Read the model definition and answer for the solid it produces. Units are mm, in the model's axes. Coordinates: 2 decimals unless noted, no trailing zeros. Write each loop counter-clockwise with the first axis right and the second up, starting at its lowest first coordinate (ties: lowest second). Pieces come first, ordered by that corner, then holes.
1) The part is cut by section A-A (z = 0). Determine the outline of the cut face in (x, y), then the cut area to 3 significant figures.
2) The part is cut by section C-C (z = -6). Determine the outline of the cut face in (x, y).
3) Determine the mould class of faces 1 (the face through (17.996, 0.986, -18.378)), 2 (the face through (-24.397, 0.986, 12.69)), 3 (the face through (-6, 2, 6)), 4 (the face through (9.63, 0.99, -17.47)) for opening direction Z: +Z half, -Z half, draft (parallel to the pull), parting line (faces both ways), or undercut.
4) Find the intervals of material crossed by line 1 (Z direction, x = -16.5, y = 0.55); line 2 (Z direction, x = -0.5, y = 1); line 3 (Z direction, x = 9, y = 1.7), in increasing order.
5) The part is cut by section B-B (x = 0). Determine the outline of the cut face in (y, z), then the cut area to 3 significant figures.
6) The part is cut by section D-D (y = 1). Give the number of separate pieces and of enclosed holes in the cut face, then the cut area to 3 significant figures.
from build123d import *

# Parameters (mm, degrees)
SKETCH_1_R           = 27.5
EXTRUDE_1_DEPTH      = 2
SKETCH_2_R           = 8
CUT_EXTRUDE_1_DEPTH  = 39.942264957
HOLE_WIZARD_M2_1_D   = 1.6
HOLE_WIZARD_M3_4_D   = 2.5
MIRROR_2_COPY_1_D    = 2.5
HOLE_WIZARD_M2_5_1_D = 2.05


with BuildPart() as part:
    # 草图1 → 凸台-拉伸1 (new body)
    with BuildSketch(Plane(origin=(0, 0, 0), x_dir=(1, 0, 0), z_dir=(0, 1, 0))):
        with Locations(Location((0, 0, 0), (0, 0, 270))):
            Circle(SKETCH_1_R)
    extrude(amount=EXTRUDE_1_DEPTH)

    # 草图2 → 切除-拉伸1 (cut, through all)
    with BuildSketch(Plane(origin=(0, 2, 0), x_dir=(1, 0, 0), z_dir=(0, 1, 0))):
        with Locations(Location((0, 0, 0), (0, 0, 270))):
            Circle(SKETCH_2_R)
    extrude(amount=-CUT_EXTRUDE_1_DEPTH, mode=Mode.SUBTRACT)

    # M2 螺纹孔1 (through all)
    with Locations(Plane(origin=(0, 2, 0), x_dir=(1, 0, 0), z_dir=(0, 1, 0))):
        with Locations((-10, 0)):
            hole_wizard_m2_1 = Hole(HOLE_WIZARD_M2_1_D / 2)

    # M3 螺纹孔4 (through all)
    with Locations(Plane(origin=(0, 2, 0), x_dir=(1, 0, 0), z_dir=(0, 1, 0))):
        with Locations((-17.324116139, 17.324116139)):
            hole_wizard_m3_4 = Hole(HOLE_WIZARD_M3_4_D / 2)

    # 镜向1: M3 螺纹孔4 across plane
    add(hole_wizard_m3_4.mirror(Plane(origin=(0, 0, 0), x_dir=(0, 0, 1), z_dir=(1, 0, 0))), mode=Mode.SUBTRACT)

    # 镜向2: M3 螺纹孔4 across plane
    add(hole_wizard_m3_4.mirror(Plane.XY), mode=Mode.SUBTRACT)

    # 镜向2 copy 1 (through all)
    with Locations(Plane(origin=(0, 2, 0), x_dir=(-1, 0, 0), z_dir=(0, 1, 0))):
        with Locations((-17.324116139, 17.324116139)):
            Hole(MIRROR_2_COPY_1_D / 2)

    # 镜向3: M2 螺纹孔1 across plane
    add(hole_wizard_m2_1.mirror(Plane(origin=(0, 0, 0), x_dir=(0, 0, 1), z_dir=(1, 0, 0))), mode=Mode.SUBTRACT)

    # M2.5 螺纹孔1 (through all)
    with Locations(Plane(origin=(0, 2, 0), x_dir=(1, 0, 0), z_dir=(0, 1, 0))):
        with Locations((-9.497088469, 16.451681088), (9.497088469, 16.451681088)):
            hole_wizard_m2_5_1 = Hole(HOLE_WIZARD_M2_5_1_D / 2)

    # 镜向4: M2.5 螺纹孔1 across plane
    add(hole_wizard_m2_5_1.mirror(Plane.XY), mode=Mode.SUBTRACT)


solid = part.part
Reported:
1. outline: (-27.5, 0) - (-10.8, 0) - (-10.8, 2) - (-27.5, 2) - close; (-9.2, 0) - (-8, 0) - (-8, 2) - (-9.2, 2) - close; (8, 0) - (9.2, 0) - (9.2, 2) - (8, 2) - close; (10.8, 0) - (27.5, 0) - (27.5, 2) - (10.8, 2) - close
1. area: 71.6 mm2
2. outline: (-26.84, 0) - (-5.29, 0) - (-5.29, 2) - (-26.84, 2) - close; (5.29, 0) - (26.84, 0) - (26.84, 2) - (5.29, 2) - close
3. face 1: undercut
3. face 2: parting line
3. face 3: draft
3. face 4: undercut
4. line 1: z = -22 to -18.26, -16.38 to 16.38, 18.26 to 22
4. line 2: z = -27.5 to -7.98, 7.98 to 27.5
4. line 3: z = -25.99 to -17.35, -15.56 to 15.56, 17.35 to 25.99
5. outline: (0, -27.5) - (2, -27.5) - (2, -8) - (0, -8) - close; (0, 8) - (2, 8) - (2, 27.5) - (0, 27.5) - close
5. area: 78.0 mm2
6. separate pieces: 1
6. enclosed holes: 11
6. area: 2,140 mm2
